from build123d import *

# Parameters (mm, degrees)
F1_DEPTH       = 6
F2_R           = 4
F3_R           = 8
F4_R           = 11
F5_R           = 1.99999
F7_D           = 3
F7_CSINK_D     = 5
F7_CSINK_ANGLE = 90


# Not quite as in the source:
# - a fillet or chamfer is up to 0.001 mm smaller than in the source, because OpenCascade refuses the exact size


with BuildPart() as f1:
    # F0 (on Front) → F1 (new body)
    with BuildSketch(Plane.XZ):
        Polygon((0, 0), (0, 20), (7, 20), (7, 24), (-4, 24), (-4, -4), (16, -4), (16, 16), (36, 16), (36, 28), (10, 28), (10, 0), align=None)
    extrude(amount=F1_DEPTH)

    # F2
    f2_edges = [f1.edges().sort_by_distance(p)[0] for p in [
        (10, -3, 0),
        (0, -3, 0),
        (0, -3, 20),
    ]]
    fillet(f2_edges, radius=F2_R)

    # F3
    f3_edges = [f1.edges().sort_by_distance(p)[0] for p in [
        (-4, -3, 24),
        (-4, -3, -4),
    ]]
    fillet(f3_edges, radius=F3_R)

    # F4
    f4_edges = [f1.edges().sort_by_distance(p)[0] for p in [
        (16, -3, -4),
    ]]
    fillet(f4_edges, radius=F4_R)

    # F5 (radius 2 in the source; OpenCascade refuses exactly that, so slightly less here)
    f5_edges = [f1.edges().sort_by_distance(p)[0] for p in [
        (7, -3, 24),
        (7, -3, 20),
    ]]
    fillet(f5_edges, radius=F5_R)

    # F7 (through all)
    with Locations(Plane(origin=(0, 0, 16), x_dir=(1, 0, 0), z_dir=(0, 0, -1))):
        with Locations((20, 3.0815127769), (31.9998442765, 3.0203789876)):
            CounterSinkHole(F7_D / 2, F7_CSINK_D / 2, counter_sink_angle=F7_CSINK_ANGLE)


solid = f1.part
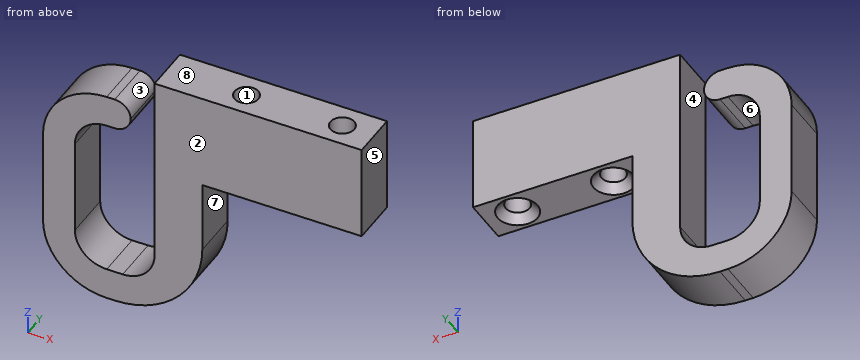
Work out the finished part from the listing and answer in its coordinate system (mm). Face numbers are marked on the shaded views. A direction names the side the tool comes from. Give positions to 0.01 mm unless a question says otherwise; leave off trailing zeros. Loops run counter-clockwise (first coordinate to the right, second up) from the corner with the lowest first, then second, coordinate; pieces in that order, holes last. Notation, with made-up numbers: M 58.5,39.5 L 100.5,39.5 A26 cw 100.5,67.5 Z; hole C 67,-26 d1. An arc over 180 degrees is marked long. Use CSV: the item, a comma, the result in double quotes.
1) Which of the six approach directions +Z, -Z, +X, -X, +Y, -Y give full straight-line access (tool end or side, diameter ignored) to the marked faces 4, 5, 6, 7 and 8?
Answer:
face 4,"+Z, +Y, -Y"
face 5,"+Z, -Z, +X, +Y, -Y"
face 6,"+Y, -Y"
face 7,"-Z, +X, +Y, -Y"
face 8,"+Z, +X, -X, +Y, -Y"
2) Find section C-C on z = 17.5. Write down the section's boundary in (x, y), plus the area to 3 significant figures.
Answer:
outline,"M -3.86,-6 L 0.29,-6 L 0.29,0 L -3.86,0 Z; M 10,-6 L 36,-6 L 36,0 L 10,0 Z; hole C 20,-3.08 d3; hole C 32,-3.02 d3"
area,"167 mm^2"
3) Find section A-A on z = 7.5. Write down the section's boundary in (x, y), plus the area to 3 significant figures.
Answer:
outline,"M -4,-6 L 0,-6 L 0,0 L -4,0 Z; M 10,-6 L 16,-6 L 16,0 L 10,0 Z"
area,"60.0 mm^2"
4) Determine the mould class of the marked faces 1, 2 and 3 for opening direction Y: released by +Y, released by -Y, zero draft, split by the parting line, or undercut.
Answer:
face 1,"undercut"
face 2,"released by -Y"
face 3,"zero draft"
5) Consider L1, parallel to X at y = -3.05, z = 24.5; L2, parallel to Y at x = 32, z = 19; L3, parallel to X at y = -4.1, z = 10. Determine where each line is inside the solid, lowest interval first.
Answer:
L1,"10 to 18.5, 21.5 to 30.5, 33.5 to 36"
L2,"-6 to -4.52, -1.52 to 0"
L3,"-4 to 0, 10 to 16"
6) Find section B-B on x = 20. Write down the section's boundary in (y, z).
Answer:
outline,"M -6,16 L -5.58,16 L -4.58,17 L -4.58,28 L -6,28 Z; M -1.58,17 L -0.58,16 L 0,16 L 0,28 L -1.58,28 Z"
7) Find section D-D on x = 2. Write down the section's boundary in (y, z), plus the area to 3 significant figures.
Answer:
outline,"M -6,-3.75 L 0,-3.75 L 0,0.54 L -6,0.54 Z; M -6,19.46 L 0,19.46 L 0,23.75 L -6,23.75 Z"
area,"51.4 mm^2"
8) Given P1, Ø1, axis at x = 5, y = -4.5, coming from the +Z side; P2, Ø2, axis at x = 25, y = -3.5, coming from the -Z side; P3, Ø1.8, axis at y = -4.5, z = 13, coming from the +X side, each flat-ended and moving along its own axis, determine where each tip first touches the part or whether it passes through.
Answer:
P1,"z = 24"
P2,"z = 16"
P3,"x = 16"
